Geometry check sheet. Reference: the model listing, model coordinates, mm. A direction names the side the tool comes from. Round coordinates to 2 decimals unless told otherwise and drop trailing zeros. Order: outer loops, then holes, each group sorted by start corner. A loop starts at its lowest first (then second) coordinate and runs counter-clockwise, first axis right, second up.
(1) Release check for a two-part mould opening along Z. For faces 4 (the face through (20, 5, -15.25)), 5 (the face through (17.875, 5, -17)), 6 (the face through (16.179, 4.93, -16.263)) record: +Z half, -Z half, draft (parallel to the pull), parting line (faces both ways), or undercut.
(2) Material ranges on line 1 along Z through (x, y) = (15.25, 7) (3 decimals); line 2 along X through (y, z) = (5.5, 16) (3 decimals); line 3 along Z through (x, y) = (-14, 5), recorded low to high.
(3) Sectioned sample at A-A (y = 5). Record the boundary of the cut face in (x, z) (3 decimals).
(4) Go/stop test with flat-tipped pins: pin 1 (1.2 mm diameter, centred on x = -20, y = 3.5, fed in from -Z); pin 2 (1.2 mm diameter, centred on x = -20.5, y = 7.5, fed in from +Z); pin 3 (2 mm diameter, centred on y = 7, z = -17, fed in from -X) (3 decimals). Record where each tip stops, or that it passes through.
(5) Sectioned sample at B-B (x = 15.25). Record the boundary of the cut face in (y, z) (3 decimals), plus the area to 3 significant figures.
(6) Set-up check for faces 1 (the face through (-17.875, 5, -17)), 2 (the face through (-17.875, 5, 17)), 3 (the face through (17.875, 5, 17)): record each of +Z, -Z, +X, -X, +Y, -Y from which the full face is reachable in a straight line by a thin tool's end or side.
from build123d import *

# Parameters (mm, degrees)
BOSS_EXTRUDE1_DEPTH     = 10
CUT_EXTRUDE1_DEPTH      = 30.970152235
CUT_EXTRUDE1_DEPTH_BACK = 30.970152235
SKETCH1_R               = 1.375


with BuildPart() as part:
    # Sketch2 → Boss-Extrude1 (new body)
    with BuildSketch(Plane(origin=(0, 0, 0), x_dir=(1, 0, 0), z_dir=(0, 1, 0))):
        Polygon((17.875, 15.25), (21.875, 15.25), (21.875, -15.25), (17.875, -15.25), (17.875, -17.88), (-17.875, -17.88), (-17.875, -15.25), (-21.875, -15.25), (-21.875, 15.25), (-17.875, 15.25), (-17.875, 17.88), (17.875, 17.88), align=None)
    extrude(amount=BOSS_EXTRUDE1_DEPTH)

    # Sketch1 → Cut-Extrude1 (cut, two sides: drawn at the far end of the back side and taken through both)
    with BuildSketch(Plane(origin=(0, 0, 0), x_dir=(1, 0, 0), z_dir=(0, 1, 0)).offset(-CUT_EXTRUDE1_DEPTH_BACK)):
        with Locations(Location((-15.25, 15.25, 0), (0, 0, 270))):
            Circle(SKETCH1_R)
        with Locations(Location((15.25, 15.25, 0), (0, 0, 270))):
            Circle(SKETCH1_R)
        with Locations(Location((15.25, -15.25, 0), (0, 0, 270))):
            Circle(SKETCH1_R)
        with Locations(Location((-15.25, -15.25, 0), (0, 0, 270))):
            Circle(SKETCH1_R)
    extrude(amount=CUT_EXTRUDE1_DEPTH + CUT_EXTRUDE1_DEPTH_BACK, mode=Mode.SUBTRACT)


solid = part.part
Answer below:
1. face 4: -Z half
1. face 5: draft
1. face 6: undercut
2. line 1: z = -17.88 to -16.625, -13.875 to 13.875, 16.625 to 17.88
2. line 2: x = -17.875 to -16.402, -14.098 to 14.098, 16.402 to 17.875
2. line 3: z = -17.88 to -15.82, -14.68 to 14.68, 15.82 to 17.88
3. outline: (-21.875, -15.25) - (-17.875, -15.25) - (-17.875, -17.88) - (17.875, -17.88) - (17.875, -15.25) - (21.875, -15.25) - (21.875, 15.25) - (17.875, 15.25) - (17.875, 17.88) - (-17.875, 17.88) - (-17.875, 15.25) - (-21.875, 15.25) - close; hole circle Ø2.75 at (-15.25, -15.25); hole circle Ø2.75 at (-15.25, 15.25); hole circle Ø2.75 at (15.25, -15.25); hole circle Ø2.75 at (15.25, 15.25)
4. pin 1: stops at z = -15.25
4. pin 2: stops at z = 15.25
4. pin 3: stops at x = -17.875
5. outline: (0, -17.88) - (10, -17.88) - (10, -16.625) - (0, -16.625) - close; (0, -13.875) - (10, -13.875) - (10, 13.875) - (0, 13.875) - close; (0, 16.625) - (10, 16.625) - (10, 17.88) - (0, 17.88) - close
5. area: 303 mm2
6. face 1: -Z, -X, +Y, -Y
6. face 2: +Z, -X, +Y, -Y
6. face 3: +Z, +X, +Y, -Y
